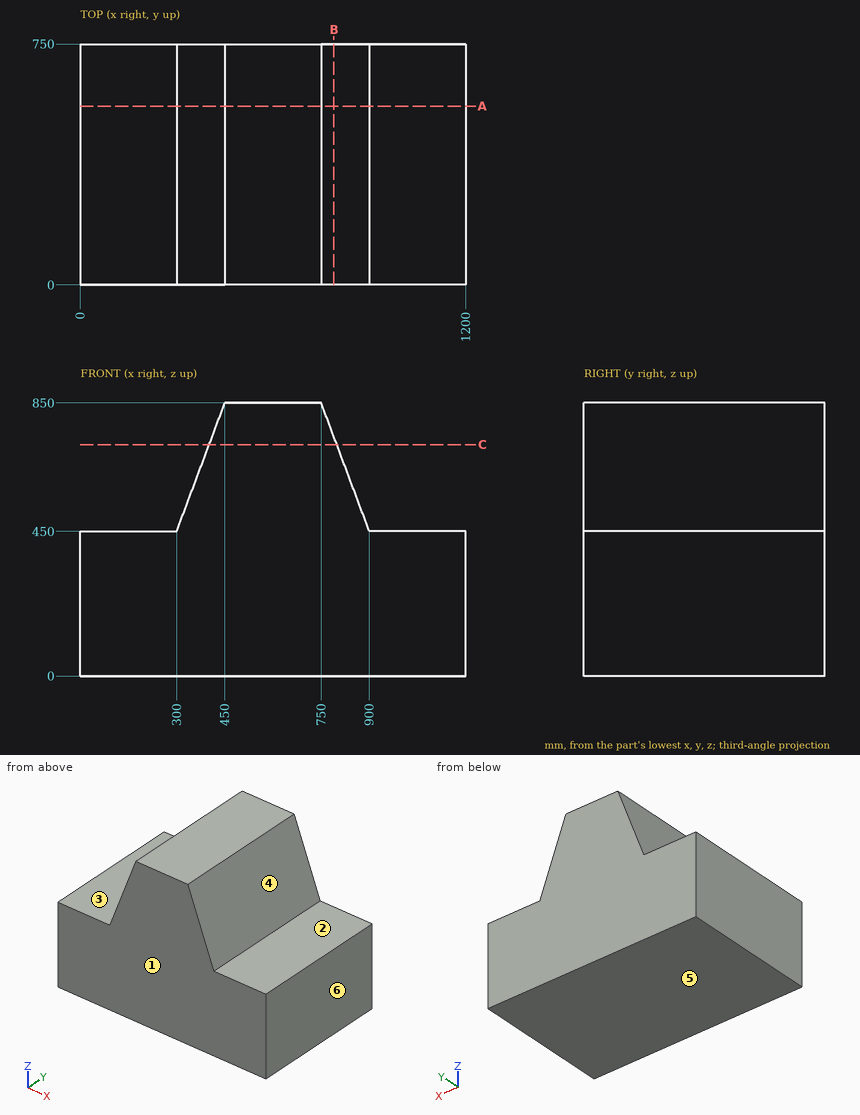
Input: dimensioned drawing with shaded views. Units: mm. Origin: part minimum x, y, z. A direction names the side the tool comes from. Coordinates: 2 decimals unless noted, no trailing zeros. Loops run counter-clockwise (first coordinate to the right, second up) from the corner with the lowest first, then second, coordinate; pieces in that order, holes last. Notation, with made-up numbers: M -25,84.25 L 14,84.25 A24 ccw 14,98.25 Z; hole C 66.25,53.5 d1. An arc over 180 degrees is marked long. Use a Markdown table: item, result. Add a question column.
1) Line query: L1, parallel to Z at x = 240, y = 90; L2, parallel to X at y = 107, z = 593.5; L3, parallel to X at y = 555, z = 464.5. Output: solid intervals per line, ascending. Write a range as from..to.
2) Set-up query: the marked faces 1, 2 and 3. Return all of +Z, -Z, +X, -X, +Y, -Y with unobstructed straight access to the full face (end or side cutting, diameter ignored); none if empty.
3) Section B-B, the plane x = 789. Return the cut outline in (y, z), plus the area to 4 significant figures.
4) Draft query along Z for the marked faces 4, 5 and 6. Return one class per face: +Z half, -Z half, draft (parallel to the pull), parting line (faces both ways), or undercut.
5) Pin query (flat end, axial travel): P1, Ø1.5, axis at y = 172, z = 696, coming from the +X side; P2, Ø1, axis at y = 317, z = 569, coming from the +X side. Return the tip coordinate at first contact, or that it passes through.
6) Section A-A, the plane y = 557. Return the cut outline in (x, z).
7) Section C-C, the plane z = 720. Return the cut outline in (x, y), plus the area to 3 significant figures.
Answer below:
| question | item | result |
|---|---|---|
| 1 | L1 | 0..450 |
| 1 | L2 | 353.81..846.19 |
| 1 | L3 | 305.44..894.56 |
| 2 | face 1 | +Z, -Z, +X, -X, -Y |
| 2 | face 2 | +Z, +X, +Y, -Y |
| 2 | face 3 | +Z, -X, +Y, -Y |
| 3 | outline | M 0,0 L 750,0 L 750,746 L 0,746 Z |
| 3 | area | 559,500 mm2 |
| 4 | face 4 | +Z half |
| 4 | face 5 | -Z half |
| 4 | face 6 | draft |
| 5 | P1 | x = 808.03 |
| 5 | P2 | x = 855.56 |
| 6 | outline | M 0,0 L 1200,0 L 1200,450 L 900,450 L 750,850 L 450,850 L 300,450 L 0,450 Z |
| 7 | outline | M 401.25,0 L 798.75,0 L 798.75,750 L 401.25,750 Z |
| 7 | area | 298,000 mm2 |
